Design review of the part built by this model. Coordinates are the model's own, in mm. A direction names the side the tool comes from. Coordinates: 2 decimals unless noted, no trailing zeros. Write each loop counter-clockwise with the first axis right and the second up, starting at its lowest first coordinate (ties: lowest second). Pieces come first, ordered by that corner, then holes. Notation, with made-up numbers: (17.25, 26) - (32.25, 26) arc R26 cw to (32.25, 61) - close; hole circle Ø10 at (57.5, 87). An arc over 180 degrees is marked (long way). Answer as a JSON object with one key per item and string values.
```python
from build123d import *

# Parameters (mm, degrees)
BASE_DEPTH        = 3.0988
SKETCH4_R         = 1.016
MOUNT_HOLES_DEPTH = 4.0988
EXTRUDE2_DEPTH    = 3.429
SKETCH3_W         = 8.382
SKETCH3_H         = 7.62
KEY_DEPTH         = 7.5278
KEYS_COUNT        = 4
KEYS_PITCH        = 14.14018
KEYS_COUNT_DIR2   = 4
KEYS_PITCH_DIR2   = 12.869418


with BuildPart() as part:
    # Sketch1 → base (new body)
    with BuildSketch(Plane.XY):
        with BuildLine():
            Line((-2.921, 31.9405), (-30.099, 31.9405))
            ThreePointArc((-30.099, 31.9405), (-31.895051224, 31.196551224), (-32.639, 29.4005))
            Line((-32.639, 29.4005), (-32.639, -29.4005))
            ThreePointArc((-32.639, -29.4005), (-31.895051224, -31.196551224), (-30.099, -31.9405))
            Line((-30.099, -31.9405), (30.099, -31.9405))
            ThreePointArc((30.099, -31.9405), (31.895051224, -31.196551224), (32.639, -29.4005))
            Line((32.639, -29.4005), (32.639, 29.4005))
            ThreePointArc((32.639, 29.4005), (31.895051224, 31.196551224), (30.099, 31.9405))
            Line((30.099, 31.9405), (2.921, 31.9405))
            Line((2.921, 31.9405), (2.921, 29.0195))
            Line((2.921, 29.0195), (-2.921, 29.0195))
            Line((-2.921, 29.0195), (-2.921, 31.9405))
        make_face()
    extrude(amount=BASE_DEPTH)

    # Sketch4 → mount holes (cut, through all)
    with BuildSketch(Plane.XY.offset(3.0988)):
        with Locations((-30, 29.5)):
            Circle(SKETCH4_R)
        with Locations((30, 29.5)):
            Circle(SKETCH4_R)
        with Locations((30, -29.5)):
            Circle(SKETCH4_R)
        with Locations((-30, -29.5)):
            Circle(SKETCH4_R)
    extrude(amount=-MOUNT_HOLES_DEPTH, mode=Mode.SUBTRACT)

    # Sketch2 → Extrude2 (add)
    with BuildSketch(Plane.XY.offset(3.0988)):
        with BuildLine():
            Line((-25.4, 28.448), (25.4, 28.448))
            ThreePointArc((25.4, 28.448), (28.632892204, 27.108892204), (29.972, 23.876))
            Line((29.972, 23.876), (29.972, -23.876))
            ThreePointArc((29.972, -23.876), (28.632892204, -27.108892204), (25.4, -28.448))
            Line((25.4, -28.448), (-25.4, -28.448))
            ThreePointArc((-25.4, -28.448), (-28.632892204, -27.108892204), (-29.972, -23.876))
            Line((-29.972, -23.876), (-29.972, 23.876))
            ThreePointArc((-29.972, 23.876), (-28.632892204, 27.108892204), (-25.4, 28.448))
        make_face()
    extrude(amount=EXTRUDE2_DEPTH)

    # Sketch3 → key (cut, through all)
    with BuildSketch(Plane.XY.offset(6.5278)):
        with Locations((-21.209, 19.304)):
            Rectangle(SKETCH3_W, SKETCH3_H)
    key = extrude(amount=-KEY_DEPTH, mode=Mode.SUBTRACT)

    # keys: key 4 × 4
    with Locations(*[(i * KEYS_PITCH, -j * KEYS_PITCH_DIR2, 0) for i in range(KEYS_COUNT) for j in range(KEYS_COUNT_DIR2) if (i, j) != (0, 0)]):
        add(key, mode=Mode.SUBTRACT)


solid = part.part
```
(1) Tool access review of faces 4 (the face through (-7, 15.494, 3)), 5 (the face through (17, 31.94, 2)), 6 (the face through (-28.67, 27.07, 4.79)): name each direction out of +Z, -Z, +X, -X, +Y, -Y from which nothing blocks a thin tool from reaching the whole face with its end or side.
Solved:
{"face 4": "+Z, -Z", "face 5": "+Z, -Z, +X, -X, +Y", "face 6": "+Z, -X, +Y"}
(2) Take a section at A-A, the plane y = -7. Write out the cut boundary in (x, z), and give its area (3 significant figures).
Solved:
{"outline": "(-32.64, 0) - (-25.4, 0) - (-25.4, 6.53) - (-29.97, 6.53) - (-29.97, 3.1) - (-32.64, 3.1) - close; (-17.02, 0) - (-11.26, 0) - (-11.26, 6.53) - (-17.02, 6.53) - close; (-2.88, 0) - (2.88, 0) - (2.88, 6.53) - (-2.88, 6.53) - close; (11.26, 0) - (17.02, 0) - (17.02, 6.53) - (11.26, 6.53) - close; (25.4, 0) - (32.64, 0) - (32.64, 3.1) - (29.97, 3.1) - (29.97, 6.53) - (25.4, 6.53) - close", "area": "189 mm^2"}
(3) Take a section at C-C, the plane x = 16. Write out the cut boundary in (y, z), and give its area (3 significant figures).
Solved:
{"outline": "(-31.94, 0) - (31.94, 0) - (31.94, 3.1) - (28.45, 3.1) - (28.45, 6.53) - (-28.45, 6.53) - (-28.45, 3.1) - (-31.94, 3.1) - close", "area": "393 mm^2"}
(4) For pin 1 (1.2 mm diameter, centred on x = -30, y = -29.5, fed in from -Z), flat-tipped, find the tip position at first contact; note if it passes through.
Solved:
{"pin 1": "passes through"}
(5) Take a section at B-B, the plane x = -18.5. Write out the cut boundary in (y, z), and give its area (3 significant figures).
Solved:
{"outline": "(-31.94, 0) - (-23.11, 0) - (-23.11, 6.53) - (-28.45, 6.53) - (-28.45, 3.1) - (-31.94, 3.1) - close; (-15.49, 0) - (-10.24, 0) - (-10.24, 6.53) - (-15.49, 6.53) - close; (-2.62, 0) - (2.62, 0) - (2.62, 6.53) - (-2.62, 6.53) - close; (10.24, 0) - (15.49, 0) - (15.49, 6.53) - (10.24, 6.53) - close; (23.11, 0) - (31.94, 0) - (31.94, 3.1) - (28.45, 3.1) - (28.45, 6.53) - (23.11, 6.53) - close", "area": "194 mm^2"}
(6) Take a section at D-D, the plane y = 27.5. Write out the cut boundary in (x, z).
Solved:
{"outline": "(-32.64, 0) - (32.64, 0) - (32.64, 3.1) - (28.19, 3.1) - (28.19, 6.53) - (-28.19, 6.53) - (-28.19, 3.1) - (-32.64, 3.1) - close"}
(7) The part is to be moulded in two halves that separate along Y. For faces 1 (the face through (0, -31.94, 2)), 2 (the face through (0, 29.02, 2)), 3 (the face through (17.021, -19, 3)), say which applies: pulls with the +Y half, pulls with the -Y half, needs draft (parallel to the pull), parting line crosses it, or undercut.
Solved:
{"face 1": "pulls with the -Y half", "face 2": "pulls with the +Y half", "face 3": "undercut"}
(8) To check wall thickness, follow line 1 (Y direction, x = 30, z = 2.05); line 2 (Y direction, x = 24, z = 4.5); line 3 (X direction, y = -17, z = 5). State the ranges of each line that lie inside material, in increasing order. Write a range as from..to.
Solved:
{"line 1": "y = -31.94..-30.52, -28.48..28.48, 30.52..31.94", "line 2": "y = -28.45..-23.11, -15.49..-10.24, -2.62..2.62, 10.24..15.49, 23.11..28.45", "line 3": "x = -29.97..-25.4, -17.02..-11.26, -2.88..2.88, 11.26..17.02, 25.4..29.97"}
